from build123d import *

# Parameters (mm, degrees)
SKETCH1_W           = 150
SKETCH1_H           = 50
BOSS_EXTRUDE1_DEPTH = 6.5
SKETCH3_R           = 5
BOSS_EXTRUDE2_DEPTH = 17.5
FILLET1_R           = 5
SKETCH4_R           = 3.2
CUT_EXTRUDE1_DEPTH  = 17.5
SKETCH5_R           = 2
CUT_EXTRUDE2_DEPTH  = 6.5


with BuildPart() as part:
    # Sketch1 → Boss-Extrude1 (new body)
    with BuildSketch(Plane(origin=(0, 0, 0), x_dir=(1, 0, 0), z_dir=(0, 1, 0))):
        Rectangle(SKETCH1_W, SKETCH1_H)
    extrude(amount=BOSS_EXTRUDE1_DEPTH)

    # Sketch3 → Boss-Extrude2 (add)
    with BuildSketch(Plane.XZ):
        with Locations(Location((45, 0, 0), (0, 0, 90))):
            Circle(SKETCH3_R)
        with Locations(Location((-45, 0, 0), (0, 0, 90))):
            Circle(SKETCH3_R)
    extrude(amount=BOSS_EXTRUDE2_DEPTH)

    # Fillet1
    fillet1_edges = [part.edges().sort_by_distance(p)[0] for p in [
        (45, 0, -5),
        (-45, 0, -5),
    ]]
    fillet(fillet1_edges, radius=FILLET1_R)

    # Sketch4 → Cut-Extrude1 (cut)
    with BuildSketch(Plane.XZ.offset(17.5)):
        with Locations(Location((45, 0, 0), (0, 0, 270))):
            Circle(SKETCH4_R)
        with Locations(Location((-45, 0, 0), (0, 0, 270))):
            Circle(SKETCH4_R)
    extrude(amount=-CUT_EXTRUDE1_DEPTH, mode=Mode.SUBTRACT)

    # Sketch5 → Cut-Extrude2 (cut)
    with BuildSketch(Plane.XZ):
        with Locations(Location((45, 0, 0), (0, 0, 270))):
            Circle(SKETCH5_R)
        with Locations(Location((-45, 0, 0), (0, 0, 270))):
            Circle(SKETCH5_R)
    extrude(amount=-CUT_EXTRUDE2_DEPTH, mode=Mode.SUBTRACT)


solid = part.part
Here's how the part is built. I have some questions about the finished solid (model axes, mm). A direction names the side the tool comes from. Coordinates: 2 decimals unless noted, no trailing zeros. Order: outer loops, then holes, each group sorted by start corner. A loop starts at its lowest first (then second) coordinate and runs counter-clockwise, first axis right, second up. Notation, with made-up numbers: (60.5, 87) -> (117.5, 87) arc R28 cw to (117.5, 105) -> close; hole circle Ø3 at (-27, 78.25). An arc over 180 degrees is marked (long way). Answer in a Markdown table with one row per item.
(1) Will this pin go through, and if not, where does the flat tip stop? pin 1 Ø3 at (x, z) = (-44.5, -1) entering from -Y.
Answer key:
| item | result |
|---|---|
| pin 1 | y = 0 |
(2) I want a section at B-B on x = -45. List the corners of the cut face in (y, z) for me, then the cut area to 3 significant figures.
Answer key:
| item | result |
|---|---|
| outline | (-17.5, -5) -> (-5, -5) arc R5 cw to (0, -10) -> (0, -25) -> (6.5, -25) -> (6.5, -2) -> (0, -2) -> (0, -3.2) -> (-17.5, -3.2) -> close; (-17.5, 3.2) -> (0, 3.2) -> (0, 2) -> (6.5, 2) -> (6.5, 25) -> (0, 25) -> (0, 10) arc R5 cw to (-5, 5) -> (-17.5, 5) -> close |
| area | 373 mm^2 |
(3) Thinking about a two-plate mould opening in X: for faces 3 (the face through (43, 0, -1)), 4 (the face through (-1, 3, 25)), 5 (the face through (-75, 3, 0)), which applies, +X half, -X half, draft (parallel to the pull), parting line (faces both ways), or undercut?
Answer key:
| item | result |
|---|---|
| face 3 | undercut |
| face 4 | draft |
| face 5 | -X half |
(4) I want a section at D-D on x = -5.5. List the corners of the cut face in (y, z) for me.
Answer key:
| item | result |
|---|---|
| outline | (0, -25) -> (6.5, -25) -> (6.5, 25) -> (0, 25) -> close |
(5) I want a section at C-C on y = -12.5. List the corners of the cut face in (x, z) for me, then the cut area to 3 significant figures.
Answer key:
| item | result |
|---|---|
| outline | circle Ø10 at (-45, 0); circle Ø10 at (45, 0); hole circle Ø6.4 at (-45, 0); hole circle Ø6.4 at (45, 0) |
| area | 92.7 mm^2 |
(6) Please list where these lines run through material, in increasing order: probe 1 along X at (y, z) = (-10.5, 0); probe 2 along Y at (x, z) = (38.5, -11).
Answer key:
| item | result |
|---|---|
| probe 1 | -50 to -48.2, -41.8 to -40, 40 to 41.8, 48.2 to 50 |
| probe 2 | 0 to 6.5 |
(7) I want a section at A-A on z = 0. Count the separate pieces of the cut face and the enclosed holes in it, then the cut area to 3 significant figures.
Answer key:
| item | result |
|---|---|
| separate pieces | 3 |
| enclosed holes | 0 |
| area | 1,070 mm^2 |
(8) On a 3-axis mill with a long thin cutter (end or side, diameter ignored), from which of +Z, -Z, +X, -X, +Y, -Y can I reach the whole of each face in a straight line? I mean faces 1 (the face through (-47, 0, -1)), 2 (the face through (48.3, -17.5, 1)). Say none if no direction works.
Answer key:
| item | result |
|---|---|
| face 1 | -Y |
| face 2 | +Z, -Z, +X, -X, -Y |
